```python
from build123d import *

# Parameters (mm, degrees)
ESQUISSE1_W             = 133.33
ESQUISSE1_H             = 160
BOSS_EXTRU_1_DEPTH      = 3
ESQUISSE2_R             = 2
ENL_V_MAT_EXTRU_1_DEPTH = 105.178799307
ESQUISSE3_R             = 2
ESQUISSE3_R_2           = 1.5
ENL_V_MAT_EXTRU_2_DEPTH = 105.178799307
ESQUISSE4_R             = 2
ENL_V_MAT_EXTRU_3_DEPTH = 3.175
ESQUISSE5_R             = 2
ENL_V_MAT_EXTRU_4_DEPTH = 105.178799307


with BuildPart() as part:
    # Esquisse1 → Boss.-Extru.1 (new body)
    with BuildSketch(Plane(origin=(0, 0, 0), x_dir=(1, 0, 0), z_dir=(0, 1, 0))):
        Rectangle(ESQUISSE1_W, ESQUISSE1_H)
    extrude(amount=BOSS_EXTRU_1_DEPTH)

    # Esquisse2 → Enlèv. mat.-Extru.1 (cut, through all)
    with BuildSketch(Plane(origin=(0, 3, 0), x_dir=(1, 0, 0), z_dir=(0, 1, 0))):
        with Locations(Location((-60.665, 74, 0), (0, 0, 270))):
            Circle(ESQUISSE2_R)
        with Locations(Location((60.665, 74, 0), (0, 0, 90))):
            Circle(ESQUISSE2_R)
        with Locations(Location((60.665, -74, 0), (0, 0, 270))):
            Circle(ESQUISSE2_R)
        with Locations(Location((-60.665, -74, 0), (0, 0, 90))):
            Circle(ESQUISSE2_R)
    extrude(amount=-ENL_V_MAT_EXTRU_1_DEPTH, mode=Mode.SUBTRACT)

    # Esquisse3 → Enlèv. mat.-Extru.2 (cut, through all)
    with BuildSketch(Plane(origin=(0, 3, 0), x_dir=(1, 0, 0), z_dir=(0, 1, 0))):
        with Locations(Location((-60.665, 27, 0), (0, 0, 270))):
            Circle(ESQUISSE3_R)
        with Locations(Location((60.665, 27, 0), (0, 0, 90))):
            Circle(ESQUISSE3_R)
        with Locations(Location((-59.165, 6.5, 0), (0, 0, 270))):
            Circle(ESQUISSE3_R_2)
        with Locations(Location((-31.165, 6.5, 0), (0, 0, 270))):
            Circle(ESQUISSE3_R_2)
        with Locations(Location((-59.165, -49, 0), (0, 0, 270))):
            Circle(ESQUISSE3_R_2)
        with Locations(Location((-31.165, -49, 0), (0, 0, 270))):
            Circle(ESQUISSE3_R_2)
        with Locations(Location((31.165, -49, 0), (0, 0, 90))):
            Circle(ESQUISSE3_R_2)
        with Locations(Location((59.165, -49, 0), (0, 0, 90))):
            Circle(ESQUISSE3_R_2)
        with Locations(Location((59.165, 6.5, 0), (0, 0, 90))):
            Circle(ESQUISSE3_R_2)
        with Locations(Location((31.165, 6.5, 0), (0, 0, 90))):
            Circle(ESQUISSE3_R_2)
    extrude(amount=-ENL_V_MAT_EXTRU_2_DEPTH, mode=Mode.SUBTRACT)

    # Esquisse4 → Enlèv. mat.-Extru.3 (cut)
    with BuildSketch(Plane(origin=(0, 3, 0), x_dir=(1, 0, 0), z_dir=(0, 1, 0))):
        with Locations(Location((-35.665, 74, 0), (0, 0, 270))):
            Circle(ESQUISSE4_R)
        with Locations(Location((35.665, 74, 0), (0, 0, 270))):
            Circle(ESQUISSE4_R)
    extrude(amount=-ENL_V_MAT_EXTRU_3_DEPTH, mode=Mode.SUBTRACT)

    # Esquisse5 → Enlèv. mat.-Extru.4 (cut, through all)
    with BuildSketch(Plane(origin=(0, 3, 0), x_dir=(1, 0, 0), z_dir=(0, 1, 0))):
        with Locations(Location((-22, 74, 0), (0, 0, 270))):
            Circle(ESQUISSE5_R)
        with Locations(Location((22, 74, 0), (0, 0, 90))):
            Circle(ESQUISSE5_R)
    extrude(amount=-ENL_V_MAT_EXTRU_4_DEPTH, mode=Mode.SUBTRACT)


solid = part.part
```
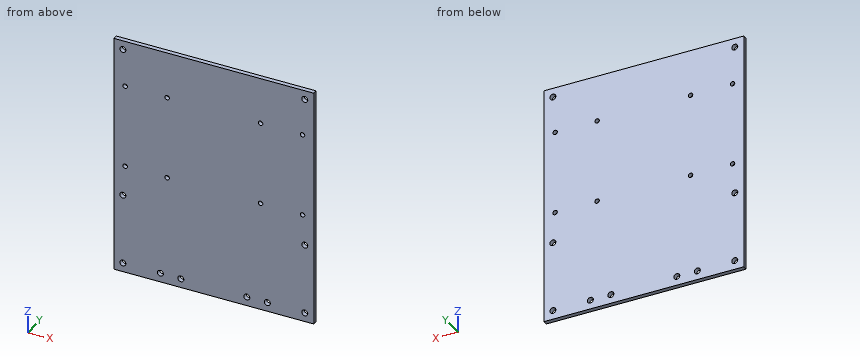
Source: CAD feature listing. Evaluate the final solid. Frame: model axes, mm. Coordinates: 2 decimals unless noted, no trailing zeros. Loops run counter-clockwise (first coordinate to the right, second up) from the corner with the lowest first, then second, coordinate; pieces in that order, holes last. Notation, with made-up numbers: (-39.75, 11) - (-2.75, 11) arc R21 ccw to (-2.75, 33) - close; hole circle Ø9 at (35.25, -36). An arc over 180 degrees is marked (long way). Answer as CSV lines item,"result".
1. Ray query, line 1 (X direction, y = 1.7, z = 49) (3 decimals); line 2 (X direction, y = 1.1, z = -7) (3 decimals); line 3 (Z direction, x = -35, y = 1.3). Return the intervals inside material, ascending.
Established:
line 1,"x = -66.665 to -60.665, -57.665 to -32.665, -29.665 to 29.665, 32.665 to 57.665, 60.665 to 66.665"
line 2,"x = -66.665 to -60.579, -57.751 to -32.579, -29.751 to 29.751, 32.579 to 57.751, 60.579 to 66.665"
line 3,"z = -80 to -75.89, -72.11 to 80"
2. Section A-A (z = -27). Return loops of the section in (x, y) (3 decimals).
Established:
outline,"(-66.665, 0) - (-62.665, 0) - (-62.665, 3) - (-66.665, 3) - close; (-58.665, 0) - (58.665, 0) - (58.665, 3) - (-58.665, 3) - close; (62.665, 0) - (66.665, 0) - (66.665, 3) - (62.665, 3) - close"
3. Section B-B (x = -22). Return loops of the section in (y, z), then the cut area to 3 significant figures.
Established:
outline,"(0, -80) - (3, -80) - (3, -76) - (0, -76) - close; (0, -72) - (3, -72) - (3, 80) - (0, 80) - close"
area,"468 mm2"
4. Contact query for a flat-ended pin moving along its axis: pin 1 (3.5 mm diameter, centred on x = 31.165, z = 49, fed in from -Y). Output: stop coordinate, or through.
Established:
pin 1,"stops at y = 0"
